from build123d import *

# Parameters (mm, degrees)
SKETCH1_R               = 5
SKETCH1_R_2             = 25
BOSS_EXTRUDE1_DEPTH     = 20
FILLET1_R               = 8
CUT_EXTRUDE4_START      = 5
CUT_EXTRUDE4_DEPTH      = 10
FILLET4_R               = 5
FILLET5_R               = 5
FILLET6_R               = 5
FILLET7_R               = 5
CUT_EXTRUDE5_DEPTH      = 68.366926205
CUT_EXTRUDE5_DEPTH_BACK = 68.366926205
SKETCH9_R               = 4
CUT_EXTRUDE6_DEPTH      = 68.366926205
CUT_EXTRUDE6_DEPTH_BACK = 68.366926205
SKETCH10_W              = 39.746236579
SKETCH10_H              = 2


with BuildPart() as part:
    # Sketch1 → Boss-Extrude1 (new body)
    with BuildSketch(Plane(origin=(0, 0, 0), x_dir=(1, 0, 0), z_dir=(0, 1, 0))):
        with BuildLine():
            ThreePointArc((13.093145751, -38.132806891), (22.75, -39.404155872), (26.47740661, -30.405400281))
            Line((26.47740661, -30.405400281), (23.370465731, -18.810139062))
            ThreePointArc((23.370465731, -18.810139062), (30, 0), (23.370465731, 18.810139062))
            Line((23.370465731, 18.810139062), (26.47740661, 30.405400281))
            ThreePointArc((26.47740661, 30.405400281), (22.75, 39.404155872), (13.093145751, 38.132806891))
            Line((13.093145751, 38.132806891), (4.604825411, 29.644486552))
            ThreePointArc((4.604825411, 29.644486552), (-17.128622381, 24.629459907), (-29.393876913, 6))
            Line((-29.393876913, 6), (-50, 6))
            Line((-50, 6), (-50, -6))
            Line((-50, -6), (-29.393876913, -6))
            ThreePointArc((-29.393876913, -6), (-17.128622381, -24.629459907), (4.604825411, -29.644486552))
            Line((4.604825411, -29.644486552), (13.093145751, -38.132806891))
        make_face()
        with Locations(Location((18.75, -32.475952642, 0), (0, 0, 270))):
            Circle(SKETCH1_R, mode=Mode.SUBTRACT)
        with Locations(Location((0, 0, 0), (0, 0, 270))):
            Circle(SKETCH1_R_2, mode=Mode.SUBTRACT)
        with Locations(Location((18.75, 32.475952642, 0), (0, 0, 270))):
            Circle(SKETCH1_R, mode=Mode.SUBTRACT)
    extrude(amount=BOSS_EXTRUDE1_DEPTH)

    # Fillet1
    fillet1_edges = [part.edges().sort_by_distance(p)[0] for p in [
        (23.370465731, 10, -18.810139062),
        (23.370465731, 10, 18.810139062),
        (4.604825411, 10, 29.644486552),
        (-29.393876913, 10, 6),
        (-29.393876913, 10, -6),
        (4.604825411, 10, -29.644486552),
    ]]
    fillet(fillet1_edges, radius=FILLET1_R)

    # Sketch8 → Cut-Extrude4 (cut)
    with BuildSketch(Plane(origin=(0, 0, 0), x_dir=(1, 0, 0), z_dir=(0, 1, 0)).offset(CUT_EXTRUDE4_START)):
        Polygon((0, 0), (112.790369841, -30.222088513), (-54.928380423, -54.928380423), align=None)
        Polygon((0, 0), (-54.928380423, 54.928380423), (112.790369841, 30.222088513), align=None)
    extrude(amount=CUT_EXTRUDE4_DEPTH, mode=Mode.SUBTRACT)

    # Fillet4
    fillet4_edges = [part.edges().sort_by_distance(p)[0] for p in [
        (-19.445436483, 5, 19.445436483),
        (-19.445436483, 15, 19.445436483),
    ]]
    fillet(fillet4_edges, radius=FILLET4_R - 0.0001)  # a hair under: the kernel refuses the full size

    # Fillet5
    fillet5_edges = [part.edges().sort_by_distance(p)[0] for p in [
        (26.562960223, 15, 7.11752374),
        (26.562960223, 5, 7.11752374),
    ]]
    fillet(fillet5_edges, radius=FILLET5_R - 0.0001)  # a hair under: the kernel refuses the full size

    # Fillet6
    fillet6_edges = [part.edges().sort_by_distance(p)[0] for p in [
        (26.562960223, 5, -7.11752374),
        (26.562960223, 15, -7.11752374),
    ]]
    fillet(fillet6_edges, radius=FILLET6_R - 0.0001)  # a hair under: the kernel refuses the full size

    # Fillet7
    fillet7_edges = [part.edges().sort_by_distance(p)[0] for p in [
        (-19.445436483, 15, -19.445436483),
        (-19.445436483, 5, -19.445436483),
    ]]
    fillet(fillet7_edges, radius=FILLET7_R - 0.0001)  # a hair under: the kernel refuses the full size

    # Sketch9 → Cut-Extrude5 (cut, two sides: drawn at the far end of the back side and taken through both)
    with BuildSketch(Plane.XY.offset(-CUT_EXTRUDE5_DEPTH_BACK)):
        with BuildLine():
            ThreePointArc((-50, 10), (-47.071067812, 17.071067812), (-40, 20))
            Line((-40, 20), (-50, 20))
            Line((-50, 20), (-50, 10))
        make_face()
        with BuildLine():
            ThreePointArc((-40, 0), (-47.071067812, 2.928932188), (-50, 10))
            Line((-50, 10), (-50, 0))
            Line((-50, 0), (-40, 0))
        make_face()
        with Locations((-40, 10)):
            Circle(SKETCH9_R)
    extrude(amount=CUT_EXTRUDE5_DEPTH + CUT_EXTRUDE5_DEPTH_BACK, mode=Mode.SUBTRACT)

    # Sketch10 → Cut-Extrude6 (cut, two sides: drawn at the far end of the back side and taken through both)
    with BuildSketch(Plane(origin=(0, 20, 0), x_dir=(1, 0, 0), z_dir=(0, 1, 0)).offset(-CUT_EXTRUDE6_DEPTH_BACK)):
        with Locations((-38.779837972, 0)):
            Rectangle(SKETCH10_W, SKETCH10_H)
    extrude(amount=CUT_EXTRUDE6_DEPTH + CUT_EXTRUDE6_DEPTH_BACK, mode=Mode.SUBTRACT)


solid = part.part
Model file for the job. Use its own axes, mm. A direction names the side the tool comes from. Give positions to 0.01 mm unless a question says otherwise; leave off trailing zeros. Order: outer loops, then holes, each group sorted by start corner. A loop starts at its lowest first (then second) coordinate and runs counter-clockwise, first axis right, second up. Notation, with made-up numbers: (45, 22) - (95, 22) arc R18 cw to (95, 45) - close; hole circle Ø8 at (76, 42). An arc over 180 degrees is marked (long way). Return JSON: item names as keys, results as strings.
1) Pull direction Y, two halves, no side cores. Call faces 4 (the flat face through (12, 15, 27)), 5 (the cylindrical face through (16.83, 2.46, -27.86)): pulls with the +Y half, pulls with the -Y half, needs draft (parallel to the pull), parting line crosses it, or undercut.
Geometry says:
{"face 4": "undercut", "face 5": "needs draft"}
2) Cut at A-A, the plane z = 15. Give the cut face in (x, y), plus the area to 3 significant figures.
Geometry says:
{"outline": "(-25.98, 0) - (-20, 0) - (-20, 20) - (-25.98, 20) - close; (20, 0) - (25.98, 0) - (25.98, 5) - (20, 5) - close; (20, 15) - (25.98, 15) - (25.98, 20) - (20, 20) - close", "area": "179 mm²"}
3) Cut at D-D, the plane x = -37. Give the cut face in (y, z).
Geometry says:
{"outline": "(0, -6) - (7.35, -6) - (7.35, -1) - (0, -1) - close; (0, 1) - (7.35, 1) - (7.35, 6) - (0, 6) - close; (12.65, -6) - (20, -6) - (20, -1) - (12.65, -1) - close; (12.65, 1) - (20, 1) - (20, 6) - (12.65, 6) - close"}
4) Cut at C-C, the plane y = 18.75. Give the cut face in (x, z).
Geometry says:
{"outline": "(-44.84, -6) - (-35.33, -6) arc R8 cw to (-27.89, -11.05) arc R30 ccw to (1.27, -29.97) arc R8 cw to (7.27, -32.31) - (13.09, -38.13) arc R8 ccw to (26.48, -30.41) - (24.35, -22.45) arc R8 cw to (25.32, -16.09) arc R30 ccw to (25.32, 16.09) arc R8 cw to (24.35, 22.45) - (26.48, 30.41) arc R8 ccw to (13.09, 38.13) - (7.27, 32.31) arc R8 cw to (1.27, 29.97) arc R30 ccw to (-27.89, 11.05) arc R8 cw to (-35.33, 6) - (-44.84, 6) - (-44.84, 1) - (-24.98, 1) arc R25 cw (long way) to (-24.98, -1) - (-44.84, -1) - close; hole circle Ø10 at (18.75, -32.48); hole circle Ø10 at (18.75, 32.48)"}
5) 3-axis set-ups, long thin cutter, end or side, ignore diameter. For faces 1 (the flat face through (-44.2, 9.9, -6)), 2 (the cylindrical face through (-18.286, 13.496, -20.302)), 3 (the flat face through (25.397, 17.465, -26.372)): which of +Z, -Z, +X, -X, +Y, -Y reach the whole face in a straight line?
Geometry says:
{"face 1": "-Z, -X, +Y, -Y", "face 2": "-Z, +X", "face 3": "+X, +Y, -Y"}
6) Cut at B-B, the plane x = 18.75. Count the separate pieces of the cut face and the enclosed holes in it, plus the area to 3 significant figures.
Geometry says:
{"separate pieces": "8", "enclosed holes": "0", "area": "279 mm²"}
7) Probe line 1 (Y direction, x = 12, z = -29); line 2 (Z direction, x = 18.75, y = 2.5); line 3 (Z direction, x = 21.5, y = 4.5). List the from-to ranges inside material, lowest first. Write a range as from..to.
Geometry says:
{"line 1": "0..5, 15..20", "line 2": "-40.48..-37.48, -27.48..-16.54, 16.54..27.48, 37.48..40.48", "line 3": "-39.99..-36.65, -28.3..-12.76, 12.76..28.3, 36.65..39.99"}
8) Flat gauge pins, fed straight in: P1, Ø8, axis at y = 3.5, z = -11, coming from the -X side; P2, Ø3, axis at x = -23, z = 22, coming from the +Y side; P3, Ø6, axis at x = -41.5, y = 14, coming from the -Z side; P4, Ø4, axis at y = 4.5, z = -22, coming from the -X side. Where does each tip first touch, or does it go through?
Geometry says:
{"P1": "x = -31.45", "P2": "through", "P3": "z = -6", "P4": "x = -22.36"}
